```python
from build123d import *

# Parameters (mm, degrees)
SKETCH1_R                = 2.2225
BAR_DEPTH                = 0.9398
SKETCH2_R                = 2.2225
CENTER_HOLE_DEPTH        = 57.878387363
OTHER_CENTER_HOLES_COUNT = 3
OTHER_CENTER_HOLES_PITCH = 12.7


with BuildPart() as part:
    # Sketch1 → Bar (new body)
    with BuildSketch(Plane(origin=(0, 0, 0), x_dir=(-1, 0, 0), z_dir=(0, 1, 0))):
        with BuildLine():
            Line((50.165, 6.35), (0, 6.35))
            ThreePointArc((0, 6.35), (-6.35, 0), (0, -6.35))
            Line((0, -6.35), (50.165, -6.35))
            ThreePointArc((50.165, -6.35), (56.515, 0), (50.165, 6.35))
        make_face()
        with Locations(Location((50.4825, 0, 0), (0, 0, 90))):
            Circle(SKETCH1_R, mode=Mode.SUBTRACT)
        with Locations(Location((-0.3175, 0, 0), (0, 0, 90))):
            Circle(SKETCH1_R, mode=Mode.SUBTRACT)
    extrude(amount=BAR_DEPTH)

    # Sketch2 → Center Hole (cut, through all)
    with BuildSketch(Plane(origin=(0, 0.9398, 0), x_dir=(1, 0, 0), z_dir=(0, 1, 0))):
        with Locations(Location((-37.7825, 0, 0), (0, 0, 270))):
            Circle(SKETCH2_R)
    center_hole = extrude(amount=-CENTER_HOLE_DEPTH, mode=Mode.SUBTRACT)

    # Other Center Holes: Center Hole ×3
    with Locations(*[(i * OTHER_CENTER_HOLES_PITCH, 0, 0) for i in range(1, OTHER_CENTER_HOLES_COUNT)]):
        add(center_hole, mode=Mode.SUBTRACT)


solid = part.part
```
Check sheet for the modelled part. Datum: model origin and axes. Units: mm. Round coordinates to 2 decimals unless told otherwise and drop trailing zeros. Write each loop counter-clockwise with the first axis right and the second up, starting at its lowest first coordinate (ties: lowest second). Pieces come first, ordered by that corner, then holes. Notation, with made-up numbers: (1.25, 37.5) -> (9.25, 37.5) arc R28 ccw to (9.25, 60.5) -> close; hole circle Ø4 at (34.5, -12.75). An arc over 180 degrees is marked (long way). Put each result on its own line as item: value.
(1) Sectioned sample at C-C (z = 4.75). Enter the section's corners in (x, y), plus the area to 3 significant figures.
Values found:
outline: (-54.38, 0) -> (4.21, 0) -> (4.21, 0.94) -> (-54.38, 0.94) -> close
area: 55.1 mm^2
(2) Mould release check, pull along Z, two halves, no side actions. Record for faces 1 (the face through (6.35, 0.46, 0.14)), 2 (the face through (-25, 0.94, 3)), 3 (the face through (-1.65, 0.46, 1.03)): released by +Z, released by -Z, zero draft, split by the parting line, or undercut.
Values found:
face 1: split by the parting line
face 2: zero draft
face 3: undercut
(3) Sectioned sample at A-A (z = 0). Enter the section's corners in (x, y) (3 decimals).
Values found:
outline: (-56.515, 0) -> (-52.705, 0) -> (-52.705, 0.94) -> (-56.515, 0.94) -> close; (-48.26, 0) -> (-40.005, 0) -> (-40.005, 0.94) -> (-48.26, 0.94) -> close; (-35.56, 0) -> (-27.305, 0) -> (-27.305, 0.94) -> (-35.56, 0.94) -> close; (-22.86, 0) -> (-14.605, 0) -> (-14.605, 0.94) -> (-22.86, 0.94) -> close; (-10.16, 0) -> (-1.905, 0) -> (-1.905, 0.94) -> (-10.16, 0.94) -> close; (2.54, 0) -> (6.35, 0) -> (6.35, 0.94) -> (2.54, 0.94) -> close
(4) Sectioned sample at B-B (y = 0.7). Count the separate pieces of the cut face and the enclosed holes in it, plus the area to 3 significant figures.
Values found:
separate pieces: 1
enclosed holes: 5
area: 686 mm^2
(5) Material ranges on line 1 (X direction, y = 0.7, z = 0) (3 decimals); line 2 (Z direction, x = -25, y = 0.3); line 3 (Z direction, x = -39, y = 0.9), recorded low to high.
Values found:
line 1: x = -56.515 to -52.705, -48.26 to -40.005, -35.56 to -27.305, -22.86 to -14.605, -10.16 to -1.905, 2.54 to 6.35
line 2: z = -6.35 to -2.22, 2.22 to 6.35
line 3: z = -6.35 to -1.86, 1.86 to 6.35
